from build123d import *

# Parameters (mm, degrees)
SKETCH1_W            = 180
SKETCH1_H            = 250
BOSS_EXTRUDE1_DEPTH  = 4
SKETCH3_W            = 180
SKETCH3_H            = 7.078404721
CUT_EXTRUDE1_DEPTH   = 2
SKETCH4_W            = 180
SKETCH4_H            = 168.5595632
BOSS_EXTRUDE3_DEPTH  = 4
CUT_EXTRUDE2_DEPTH   = 214
SKETCH6_W            = 4
SKETCH6_H            = 40
BOSS_EXTRUDE4_DEPTH  = 25
SKETCH7_W            = 80
SKETCH7_H            = 50
CUT_EXTRUDE3_DEPTH   = 5
SKETCH8_R            = 1.4
CUT_EXTRUDE4_DEPTH   = 155
SKETCH10_W           = 50
SKETCH10_H           = 6.222895308
BOSS_EXTRUDE5_DEPTH  = 10
CUT_EXTRUDE5_DEPTH   = 199
SKETCH12_W           = 20
SKETCH12_H           = 200
CUT_EXTRUDE6_DEPTH   = 5
SKETCH13_R           = 5
SKETCH13_R_2         = 1.6
BOSS_EXTRUDE6_DEPTH  = 30
SKETCH14_R           = 4.6
SKETCH14_R_2         = 1.6
BOSS_EXTRUDE7_DEPTH  = 15
BOSS_EXTRUDE8_DEPTH  = 4
BOSS_EXTRUDE9_DEPTH  = 4
SKETCH17_W           = 25
SKETCH17_H           = 70
CUT_EXTRUDE8_DEPTH   = 19
SKETCH18_R           = 4
CUT_EXTRUDE9_DEPTH   = 145
BOSS_EXTRUDE10_DEPTH = 180
SKETCH27_W           = 80
SKETCH27_H           = 3.378884896
BOSS_EXTRUDE17_DEPTH = 3
BOSS_EXTRUDE13_DEPTH = 3
BOSS_EXTRUDE14_DEPTH = 3
BOSS_EXTRUDE15_DEPTH = 3
BOSS_EXTRUDE16_DEPTH = 3
FILLET1_R            = 1
SKETCH28_W           = 80
SKETCH28_H           = 34.31128583
CUT_EXTRUDE14_DEPTH  = 3


with BuildPart() as part:
    # Sketch1 → Boss-Extrude1 (new body)
    with BuildSketch(Plane(origin=(0, 0, 0), x_dir=(1, 0, 0), z_dir=(0, 1, 0))):
        with Locations((90, 125)):
            Rectangle(SKETCH1_W, SKETCH1_H)
    extrude(amount=BOSS_EXTRUDE1_DEPTH)

    # Sketch3 → Cut-Extrude1 (cut)
    with BuildSketch(Plane(origin=(0, 124.753672771, -148.675637714), x_dir=(-1, 0, 0), z_dir=(0, 0.6427876096865376, -0.7660444431189795))):
        with Locations((-90, -157.157700062)):
            Rectangle(SKETCH3_W, SKETCH3_H)
    extrude(amount=-CUT_EXTRUDE1_DEPTH, mode=Mode.SUBTRACT)

    # Sketch4 → Boss-Extrude3 (add)
    with BuildSketch(Plane(origin=(0, 123.468097552, -147.143548828), x_dir=(-1, 0, 0), z_dir=(0, 0.6427876096865368, -0.7660444431189802))):
        with Locations((-90, -133.637022031)):
            Rectangle(SKETCH4_W, SKETCH4_H)
    extrude(amount=BOSS_EXTRUDE3_DEPTH)

    # Sketch5 → Cut-Extrude2 (cut)
    with BuildSketch(Plane.ZY):
        Polygon((-287.217770145, -43.465858932), (-287.217770145, -37.242963624), (-290.281947917, -40.894708493), align=None)
    extrude(amount=-CUT_EXTRUDE2_DEPTH, mode=Mode.SUBTRACT)

    # Sketch6 → Boss-Extrude4 (add)
    with BuildSketch(Plane.XZ):
        with Locations((29, -203.745583946)):
            Rectangle(SKETCH6_W, SKETCH6_H)
        with Locations((29, -35)):
            Rectangle(SKETCH6_W, SKETCH6_H)
        with Locations((151, -203.745583946)):
            Rectangle(SKETCH6_W, SKETCH6_H)
        with Locations((151, -35)):
            Rectangle(SKETCH6_W, SKETCH6_H)
    extrude(amount=BOSS_EXTRUDE4_DEPTH)

    # Sketch7 → Cut-Extrude3 (cut)
    with BuildSketch(Plane(origin=(0, 126.039247991, -150.207726601), x_dir=(-1, 0, 0), z_dir=(0, 0.6427876096865365, -0.7660444431189805))):
        with Locations((-90, -192.916803631)):
            Rectangle(SKETCH7_W, SKETCH7_H)
        Polygon((-150, -49.357240431), (-107.5, -113.87549192), (-72.5, -113.87549192), (-30, -49.357240431), align=None)
    extrude(amount=-CUT_EXTRUDE3_DEPTH, mode=Mode.SUBTRACT)

    # Sketch8 → Cut-Extrude4 (cut)
    with BuildSketch(Plane.ZY.offset(-27)):
        with Locations((-187.745583946, -2.5)):
            Circle(SKETCH8_R)
        with Locations((-187.745583946, -20)):
            Circle(SKETCH8_R)
        with Locations((-51, -2.5)):
            Circle(SKETCH8_R)
        with Locations((-51, -20)):
            Circle(SKETCH8_R)
    extrude(amount=-CUT_EXTRUDE4_DEPTH, mode=Mode.SUBTRACT)

    # Sketch10 → Boss-Extrude5 (add)
    with BuildSketch(Plane(origin=(0, 0, -287.217770145), x_dir=(-1, 0, 0), z_dir=(0, 0, -1))):
        with Locations((-155, -40.354411278)):
            Rectangle(SKETCH10_W, SKETCH10_H)
        with Locations((-25, -40.354411278)):
            Rectangle(SKETCH10_W, SKETCH10_H)
    extrude(amount=BOSS_EXTRUDE5_DEPTH)

    # Sketch11 → Cut-Extrude5 (cut)
    with BuildSketch(Plane.ZY):
        Polygon((-297.217770145, -41.965858932), (-287.217770145, -37.242963624), (-297.217770145, -37.242963624), align=None)
    extrude(amount=-CUT_EXTRUDE5_DEPTH, mode=Mode.SUBTRACT)

    # Sketch12 → Cut-Extrude6 (cut)
    with BuildSketch(Plane(origin=(0, 4, 0), x_dir=(1, 0, 0), z_dir=(0, 1, 0))):
        with Locations((90, 130)):
            Rectangle(SKETCH12_W, SKETCH12_H)
    extrude(amount=-CUT_EXTRUDE6_DEPTH, mode=Mode.SUBTRACT)

    # Sketch13 → Boss-Extrude6 (add)
    # profile 1 of 4: a face of its own
    with BuildSketch(Plane(origin=(0, 4, 0), x_dir=(1, 0, 0), z_dir=(0, 1, 0))):
        with Locations(Location((64.5, 99.1, 0), (0, 0, 90))):
            Circle(SKETCH13_R)
        with Locations(Location((64.5, 99.1, 0), (0, 0, 270))):
            Circle(SKETCH13_R_2, mode=Mode.SUBTRACT)
    # profile 2 of 4: a face of its own
    with BuildSketch(Plane(origin=(0, 4, 0), x_dir=(1, 0, 0), z_dir=(0, 1, 0))):
        with Locations(Location((115.5, 99.1, 0), (0, 0, 90))):
            Circle(SKETCH13_R)
        with Locations(Location((115.5, 99.1, 0), (0, 0, 270))):
            Circle(SKETCH13_R_2, mode=Mode.SUBTRACT)
    # profile 3 of 4: a face of its own
    with BuildSketch(Plane(origin=(0, 4, 0), x_dir=(1, 0, 0), z_dir=(0, 1, 0))):
        with Locations(Location((115.5, 20, 0), (0, 0, 90))):
            Circle(SKETCH13_R)
        with Locations(Location((115.5, 20, 0), (0, 0, 270))):
            Circle(SKETCH13_R_2, mode=Mode.SUBTRACT)
    # profile 4 of 4: a face of its own
    with BuildSketch(Plane(origin=(0, 4, 0), x_dir=(1, 0, 0), z_dir=(0, 1, 0))):
        with Locations(Location((64.5, 20, 0), (0, 0, 90))):
            Circle(SKETCH13_R)
        with Locations(Location((64.5, 20, 0), (0, 0, 270))):
            Circle(SKETCH13_R_2, mode=Mode.SUBTRACT)
    extrude(amount=BOSS_EXTRUDE6_DEPTH)

    # Sketch14 → Boss-Extrude7 (add)
    # profile 1 of 8: a face of its own
    with BuildSketch(Plane(origin=(0, 4, 0), x_dir=(1, 0, 0), z_dir=(0, 1, 0))):
        with Locations(Location((32, 166.671215293, 0), (0, 0, 90))):
            Circle(SKETCH14_R)
        with Locations(Location((32, 166.671215293, 0), (0, 0, 270))):
            Circle(SKETCH14_R_2, mode=Mode.SUBTRACT)
    # profile 2 of 8: a face of its own
    with BuildSketch(Plane(origin=(0, 4, 0), x_dir=(1, 0, 0), z_dir=(0, 1, 0))):
        with Locations(Location((72, 166.671215293, 0), (0, 0, 90))):
            Circle(SKETCH14_R)
        with Locations(Location((72, 166.671215293, 0), (0, 0, 270))):
            Circle(SKETCH14_R_2, mode=Mode.SUBTRACT)
    # profile 3 of 8: a face of its own
    with BuildSketch(Plane(origin=(0, 4, 0), x_dir=(1, 0, 0), z_dir=(0, 1, 0))):
        with Locations(Location((72, 126.671215293, 0), (0, 0, 90))):
            Circle(SKETCH14_R)
        with Locations(Location((72, 126.671215293, 0), (0, 0, 270))):
            Circle(SKETCH14_R_2, mode=Mode.SUBTRACT)
    # profile 4 of 8: a face of its own
    with BuildSketch(Plane(origin=(0, 4, 0), x_dir=(1, 0, 0), z_dir=(0, 1, 0))):
        with Locations(Location((32, 126.671215293, 0), (0, 0, 90))):
            Circle(SKETCH14_R)
        with Locations(Location((32, 126.671215293, 0), (0, 0, 270))):
            Circle(SKETCH14_R_2, mode=Mode.SUBTRACT)
    # profile 5 of 8: a face of its own
    with BuildSketch(Plane(origin=(0, 4, 0), x_dir=(1, 0, 0), z_dir=(0, 1, 0))):
        with Locations(Location((108, 166.671215293, 0), (0, 0, 90))):
            Circle(SKETCH14_R)
        with Locations(Location((108, 166.671215293, 0), (0, 0, 270))):
            Circle(SKETCH14_R_2, mode=Mode.SUBTRACT)
    # profile 6 of 8: a face of its own
    with BuildSketch(Plane(origin=(0, 4, 0), x_dir=(1, 0, 0), z_dir=(0, 1, 0))):
        with Locations(Location((148, 166.671215293, 0), (0, 0, 90))):
            Circle(SKETCH14_R)
        with Locations(Location((148, 166.671215293, 0), (0, 0, 270))):
            Circle(SKETCH14_R_2, mode=Mode.SUBTRACT)
    # profile 7 of 8: a face of its own
    with BuildSketch(Plane(origin=(0, 4, 0), x_dir=(1, 0, 0), z_dir=(0, 1, 0))):
        with Locations(Location((148, 126.671215293, 0), (0, 0, 90))):
            Circle(SKETCH14_R)
        with Locations(Location((148, 126.671215293, 0), (0, 0, 270))):
            Circle(SKETCH14_R_2, mode=Mode.SUBTRACT)
    # profile 8 of 8: a face of its own
    with BuildSketch(Plane(origin=(0, 4, 0), x_dir=(1, 0, 0), z_dir=(0, 1, 0))):
        with Locations(Location((108, 126.671215293, 0), (0, 0, 90))):
            Circle(SKETCH14_R)
        with Locations(Location((108, 126.671215293, 0), (0, 0, 270))):
            Circle(SKETCH14_R_2, mode=Mode.SUBTRACT)
    extrude(amount=BOSS_EXTRUDE7_DEPTH)

    # Sketch15 → Boss-Extrude8 (add)
    with BuildSketch(Plane.ZY.offset(-30)):
        Polygon((0, 4), (0, 80.750364276), (-19.301891028, 80.750364276), (-87.419317565, 4), (-67.363636364, 4), (-15, 63), (-15, 4), align=None)
    boss_extrude8 = extrude(amount=BOSS_EXTRUDE8_DEPTH)

    # Mirror1: Boss-Extrude8 across plane
    add(boss_extrude8.mirror(Plane(origin=(90, 0, 0), x_dir=(0, 0, 1), z_dir=(1, 0, 0))))

    # Sketch16 → Boss-Extrude9 (add)
    with BuildSketch(Plane.ZY.offset(-30)):
        Polygon((-212.271069219, 45.852141149), (-212.271069219, 4), (-204.271069219, 4), (-204.271069219, 55.38616989), align=None)
        Polygon((-234.18477544, 19.736403034), (-234.18477544, 4), (-226.18477544, 4), (-226.18477544, 29.270431775), align=None)
    boss_extrude9 = extrude(amount=BOSS_EXTRUDE9_DEPTH)

    # Mirror2: Boss-Extrude9 across plane
    add(boss_extrude9.mirror(Plane(origin=(90, 0, 0), x_dir=(0, 0, 1), z_dir=(1, 0, 0))))

    # Sketch17 → Cut-Extrude8 (cut)
    with BuildSketch(Plane(origin=(0, 4, 0), x_dir=(1, 0, 0), z_dir=(0, 1, 0))):
        with Locations((12.5, 35)):
            Rectangle(SKETCH17_W, SKETCH17_H)
        with Locations((12.5, 206.553921427)):
            Rectangle(SKETCH17_W, SKETCH17_H)
    cut_extrude8 = extrude(amount=-CUT_EXTRUDE8_DEPTH, mode=Mode.SUBTRACT)

    # Sketch18 → Cut-Extrude9 (cut)
    with BuildSketch(Plane.ZY.offset(-27)):
        with Locations((-29.5, -11.2)):
            Circle(SKETCH18_R)
        with Locations((-209.245583946, -11.2)):
            Circle(SKETCH18_R)
    extrude(amount=-CUT_EXTRUDE9_DEPTH, mode=Mode.SUBTRACT)

    # Mirror3: Cut-Extrude8 across plane
    add(cut_extrude8.mirror(Plane(origin=(90, 0, 0), x_dir=(0, 0, 1), z_dir=(1, 0, 0))), mode=Mode.SUBTRACT)



with BuildPart() as body_2:
    # Sketch19 → Boss-Extrude10 (new body)
    with BuildSketch(Plane.ZY):
        Polygon((-250, 0.888552346), (-250, -43.052683021), (-287.710174021, -43.052683021), (-284.353775496, -40.052683021), (-252.906484315, -40.052683021), (-252.906484315, -2.575260778), align=None)
    extrude(amount=-BOSS_EXTRUDE10_DEPTH)


with BuildPart() as part_1:
    add(part.part)

    add(body_2.part)  # Boss-Extrude17 merges body 2
    # Sketch27 → Boss-Extrude17 (add)
    with BuildSketch(Plane(origin=(0, 123.468097552, -147.143548828), x_dir=(-1, 0, 0), z_dir=(0, 0.6427876096865226, -0.766044443118992))):
        with Locations((-90, -166.227361183)):
            Rectangle(SKETCH27_W, SKETCH27_H)
    extrude(amount=BOSS_EXTRUDE17_DEPTH)

    # Sketch23 → Boss-Extrude13 (add)
    with BuildSketch(Plane(origin=(50, 0, 0), x_dir=(0, 0, -1), z_dir=(1, 0, 0))):
        Polygon((250, 0.888552346), (287.710174021, -43.052683021), (250, -43.052683021), align=None)
    extrude(amount=-BOSS_EXTRUDE13_DEPTH)

    # Sketch24 → Boss-Extrude14 (add)
    with BuildSketch(Plane.ZY.offset(-130)):
        Polygon((-252.906484315, -2.575260778), (-252.906484315, -40.052683021), (-284.353775496, -40.052683021), align=None)
    extrude(amount=-BOSS_EXTRUDE14_DEPTH)

    # Sketch25 → Boss-Extrude15 (add)
    with BuildSketch(Plane.ZY):
        Polygon((-252.906484315, -2.575260778), (-252.906484315, -40.052683021), (-284.353775496, -40.052683021), align=None)
    extrude(amount=-BOSS_EXTRUDE15_DEPTH)

    # Sketch26 → Boss-Extrude16 (add)
    with BuildSketch(Plane(origin=(180, 0, 0), x_dir=(0, 0, -1), z_dir=(1, 0, 0))):
        Polygon((252.906484315, -2.575260778), (252.906484315, -40.052683021), (284.353775496, -40.052683021), align=None)
    extrude(amount=-BOSS_EXTRUDE16_DEPTH)

    # Fillet1
    fillet1_edges = [part_1.edges().sort_by_distance(p)[0] for p in [
        (90, -43.052683021, -250),
    ]]
    fillet(fillet1_edges, radius=FILLET1_R)

    # Sketch28 → Cut-Extrude14 (cut)
    with BuildSketch(Plane(origin=(0, -40.052683021, 0), x_dir=(1, 0, 0), z_dir=(0, 1, 0))):
        with Locations((90, 270.06212723)):
            Rectangle(SKETCH28_W, SKETCH28_H)
    extrude(amount=-CUT_EXTRUDE14_DEPTH, mode=Mode.SUBTRACT)


solid = part_1.part
Could you check a few things on this model? Use its own coordinates, in mm. A direction names the side the tool comes from. Coordinates: 2 decimals unless noted, no trailing zeros. Loops run counter-clockwise (first coordinate to the right, second up) from the corner with the lowest first, then second, coordinate; pieces in that order, holes last.
1. Imagine slicing it at A-A (x = 164). Please give me the cut outline in (y, z).
2. We'd pull the mould along Z, two halves only. Please class faces 5 (the face through (24.65, -39.64, -292.29)), 6 (the face through (34, 19, -127)), 7 (the face through (88.7, -43.053, -252.7)): released by +Z, released by -Z, zero draft, split by the parting line, or undercut.
3. Imagine slicing it at B-B (x = 56). Please give me the cut outline in (y, z), and give its area (3 significant figures).
4. I need wall thicknesses on L1, parallel to X at y = 15, z = -99; L2, parallel to Z at x = 115, y = 24; L3, parallel to X at y = 57, z = -24.5. Which ranges of each line are inside material? Lowest first, please.
5. For faces 1 (the face through (150, 45, -34)), 2 (the face through (153, -12, -35)), 3 (the face through (3, -29, -261)), 4 (the face through (31, -12, -204)), which set-ups out of +Z, -Z, +X, -X, +Y, -Y let a thin tool reach every point of the face, with its end or its side?
6. Imagine slicing it at C-C (y = 74.5). Please give me the cut outline in (x, z), and give its area (3 significant figures).
7. For P1, Ø2.5, axis at y = 30, z = -209, coming from the +X side; P2, Ø1.2, axis at x = 153, y = 10, coming from the -Z side; P3, Ø5, axis at y = -22.5, z = -44.5, coming from the +X side, each with a flat end and sliding along its axis, tell me the tip position at first contact or that it passes through.
Computed values:
1. outline: (-43.47, -297.22) - (-41.97, -297.22) - (-37.24, -287.22) - (88.23, -181.93) - (85.66, -178.87) - (4, -247.39) - (4, -241.55) - (0, -241.55) - (0, -250) - (-42.05, -250) arc R1 ccw to (-43.05, -251) - (-43.05, -286.87) - (-43.47, -287.22) - close; (0, -171.55) - (4, -171.55) - (4, -70) - (0, -70) - close; hole (-40.05, -284.35) - (-2.58, -252.91) - (-40.05, -252.91) - close
2. face 5: released by -Z
2. face 6: undercut
2. face 7: zero draft
3. outline: (-43.05, -287.71) - (-42.61, -287.22) - (-43.05, -287.22) - close; (-43.05, -252.91) - (-2.58, -252.91) - (-5.16, -255.08) - (-2.59, -258.14) - (57.99, -207.3) - (55.42, -204.24) - (4, -247.39) - (4, 0) - (0, 0) - (0, -250) - (-42.05, -250) arc R1 ccw to (-43.05, -251) - close
3. area: 1,430 mm2
4. L1: x = 59.5 to 62.9, 66.1 to 69.5, 110.5 to 113.9, 117.1 to 120.5
4. L2: z = -235.83 to -230.61, -104.07 to -100.62, -97.58 to -94.13, -24.97 to -21.52, -18.48 to -15.03
4. L3: x = 26 to 30, 150 to 154
5. face 1: +Z, +Y
5. face 2: +Z, +X, -Y
5. face 3: none
5. face 4: +Z, -Y
6. outline: (0, -193.45) - (41.81, -193.45) - (39.6, -188.23) - (0, -188.23) - close; (26, -24.85) - (30, -24.85) - (30, 0) - (26, 0) - close; (138.19, -193.45) - (180, -193.45) - (180, -188.23) - (140.4, -188.23) - close; (150, -24.85) - (154, -24.85) - (154, 0) - (150, 0) - close
6. area: 624 mm2
7. P1: stops at x = 154
7. P2: stops at z = -248.08
7. P3: stops at x = 153
